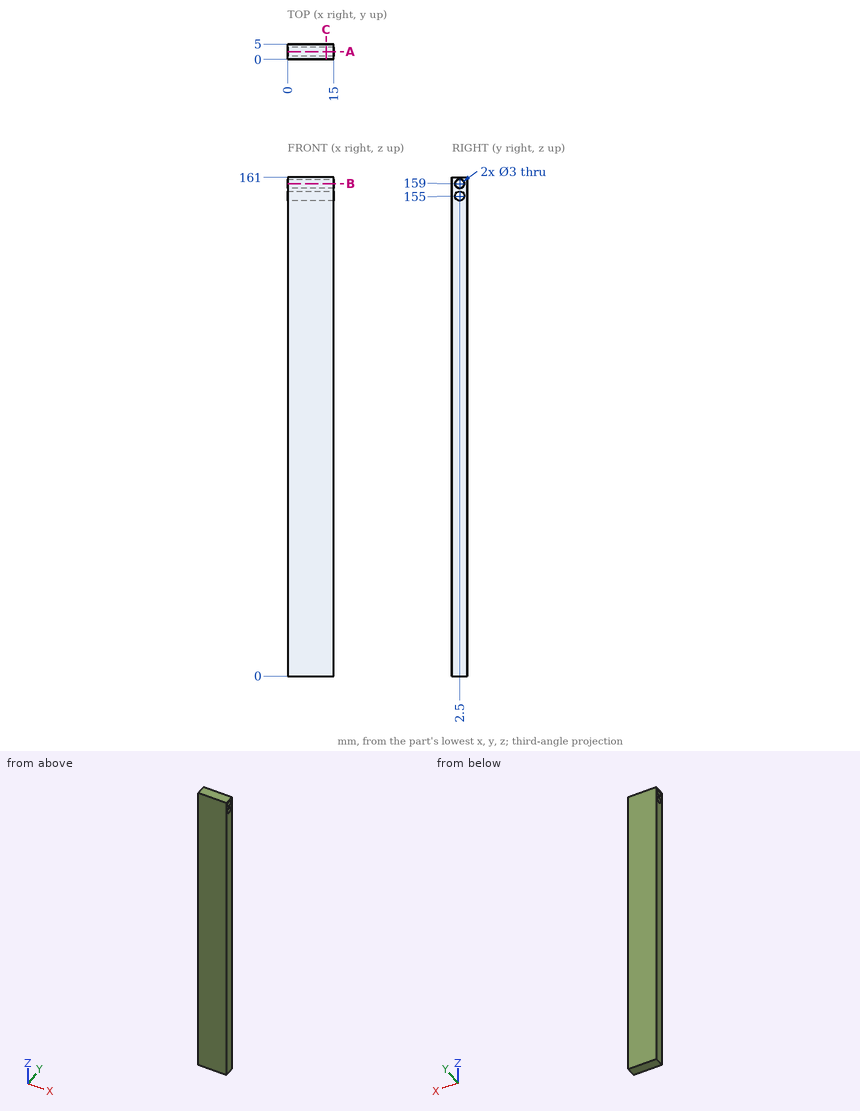
For this review, use the dimensioned drawing (mm, ordinates from the lowest corner) and the shaded views. Round coordinates to 2 decimals unless told otherwise and drop trailing zeros. Write each loop counter-clockwise with the first axis right and the second up, starting at its lowest first coordinate (ties: lowest second). Pieces come first, ordered by that corner, then holes. Notation, with made-up numbers: (-15.75, -31) -> (37.25, -31) arc R27 cw to (37.25, -6) -> close; hole circle Ø6 at (66, 65.25). An arc over 180 degrees is marked (long way). One line per item, written item: value. Start each with the question number.
Q1. Add section B-B (z = 159). Give the boundary of the cut face in (x, y), then the cut area to 3 significant figures.
Q2. To check wall thickness, follow probe 1 along Z at (x, y) = (3, 2.4); probe 2 along Y at (x, z) = (7.5, 159); probe 3 along Z at (x, y) = (9.25, 3.75). State the ranges of each line that lie inside material, in increasing order.
Q3. Add section C-C (x = 12.5). Give the boundary of the cut face in (y, z), then the cut area to 3 significant figures.
Q4. Add section A-A (y = 2.5). Give the boundary of the cut face in (x, z), then the cut area to 4 significant figures.
Response:
1. outline: (0, 0) -> (15, 0) -> (15, 1) -> (0, 1) -> close; (0, 4) -> (15, 4) -> (15, 5) -> (0, 5) -> close
1. area: 30.0 mm^2
2. probe 1: z = 0 to 153.5, 156.5 to 157.5, 160.5 to 161
2. probe 2: y = 0 to 1, 4 to 5
2. probe 3: z = 0 to 154.17, 155.83 to 158.17, 159.83 to 161
3. outline: (0, 0) -> (5, 0) -> (5, 161) -> (0, 161) -> close; hole circle Ø3 at (2.5, 155); hole circle Ø3 at (2.5, 159)
3. area: 791 mm^2
4. outline: (0, 0) -> (15, 0) -> (15, 153.5) -> (0, 153.5) -> close; (0, 156.5) -> (15, 156.5) -> (15, 157.5) -> (0, 157.5) -> close; (0, 160.5) -> (15, 160.5) -> (15, 161) -> (0, 161) -> close
4. area: 2,325 mm^2
